Autodesk Inventor part; units mm, degrees
ref_plane "YZ Plane" through (0, 0, 0) normal (1, 0, 0) x (0, 1, 0)
ref_plane "XZ Plane" through (0, 0, 0) normal (0, 1, 0) x (-1, 0, 0)
ref_plane "XY Plane" through (0, 0, 0) normal (0, 0, 1) x (1, 0, 0)
sketch "Sketch1" plane through (0, 0, 0) normal (0, 1, 0) x (-1, 0, 0)
  line L0 (0, 0) -> (10.922, 0)
  line L1 (10.922, 0) -> (10.922, 203.2)
  line L2 (10.922, 203.2) -> (0, 203.2)
  line L3 (0, 203.2) -> (0, 0)
  line L4 (10.922, 203.2) -> (-166.878, 203.2)
  line L5 (-166.878, 203.2) -> (-166.878, 181.102)
  line L6 (-166.878, 181.102) -> (10.922, 181.102)
  line L7 (10.922, 181.102) -> (10.922, 203.2)
  point P0 (0, 181.102)
  dimension "d0" = 10.922
  dimension "d1" = 203.2
  dimension "d16" = 177.8
  dimension "d17" = 22.098
extrude "Extrusion1" add sketch "Sketch1" along normal blind 50.8
sketch "Sketch3" plane through (0, 0, 181.102) normal (1, 0, 0) x (0, 0, -1)
  circle A0 centre (28.702, 25.4) radius 2.5797
  circle A1 centre (130.302, 25.4) radius 2.5797
  line L0 (181.102, 0) -> (181.102, 50.8)
  line L1 (0, 0) -> (181.102, 0)
  circle A2 centre (130.302, 25.4) radius 3.9688
  circle A3 centre (28.702, 25.4) radius 3.9687
  dimension "d18" = 5.1594
  dimension "d19" = 5.1594
  dimension "d20" = 0
  dimension "d21" = 101.6
  dimension "d22" = 50.8
  dimension "d23" = 25.4
  dimension "d24" = 7.9375
  dimension "d25" = 7.9375
sketch "Sketch4" plane through (166.878, 0, 181.102) normal (0, 0, -1) x (-1, 0, 0)
  circle A0 centre (50.8, 25.4) radius 2.5797
  circle A1 centre (127, 25.4) radius 2.5797
  line L0 (0, 0) -> (0, 50.8)
  circle A2 centre (50.8, 25.4) radius 3.9687
  circle A3 centre (127, 25.4) radius 3.9687
  line L1 (0, 0) -> (166.878, 0)
  dimension "d26" = 5.1594
  dimension "d27" = 5.1594
  dimension "d28" = 0
  dimension "d29" = 76.2
  dimension "d30" = 50.8
  dimension "d31" = 7.9375
  dimension "d32" = 7.9375
  dimension "d33" = 25.4
extrude "Extrusion4" cut sketch "Sketch4" against normal through all contours A0 | A1
extrude "Extrusion5" cut sketch "Sketch4" against normal blind 5.1594 contours A0 | A1 | A2 | A3
extrude "Extrusion6" cut sketch "Sketch3" against normal blind 5.1594 contours A0 | A1 | A2 | A3
extrude "Extrusion7" cut sketch "Sketch3" against normal through all contours A0 | A1
equation "\"d19\" = d18"
equation "\"d26\" = d18"
equation "\"d27\" = d26"
equation "\"d31\" = d24"
equation "\"d32\" = d31"
properties part number "battery shim"
The listing builds one solid part. Answer for the finished solid, in the listing's coordinates (mm). A direction names the side the tool comes from. Coordinates: 2 decimals unless noted, no trailing zeros. Write each loop counter-clockwise with the first axis right and the second up, starting at its lowest first coordinate (ties: lowest second). Pieces come first, ordered by that corner, then holes. Notation, with made-up numbers: (-20, 77.5) - (1, 77.5) arc R21 cw to (1, 86.5) - close; hole circle Ø9 at (25, 34.5). An arc over 180 degrees is marked (long way). Return JSON: item names as keys, results as strings. Group by question number.
1. Straight lines are drawn through the part: L1, parallel to Z at x = -2, y = 25; L2, parallel to X at y = 25, z = 184; L3, parallel to X at y = 25, z = 199. For each, find the intervals that lie inside material, in ascending order.
2. A cutting plane is placed at A-A, the plane z = 50.8. Determine the outline of the cut face in (x, y).
3. Which of the six approach directions +Z, -Z, +X, -X, +Y, -Y give full straight-line access (tool end or side, diameter ignored) to faces 4 (the flat face through (-5, 25, 0)), 5 (the cylindrical face through (118.655, 25.513, 194.612)), 6 (the flat face through (85, 25, 181.102)), 7 (the cylindrical face through (-2.544, 25.575, 54.765)), 8 (the flat face through (113, 25, 186.261))?
4. A cutting plane is placed at D-D, the plane y = 44.5. Determine the outline of the cut face in (x, z), plus the area to 3 significant figures.
5. Given pin 1 (6 mm diameter, centred on y = 25.4, z = 152.4, fed in from +X); pin 2 (6 mm diameter, centred on x = 39.878, y = 25.4, fed in from -Z); pin 3 (15 mm diameter, centred on x = 115.5, y = 27.5, fed in from -Z), each flat-ended and moving along its own axis, determine where each tip first touches the part or whether it passes through.
6. Determine the mould class of faces 1 (the flat face through (45, 50.8, 185)), 2 (the flat face through (0, 25, 92)), 3 (the cylindrical face through (37.5, 24.4, 194.6)) for opening direction X: released by +X, released by -X, zero draft, split by the parting line, or undercut.
7. A cutting plane is placed at C-C, the plane y = 25.4. Give the number of separate pieces and of enclosed holes in the cut face, plus the area to 3 significant figures.
Ans:
{
 "1": {"L1": "0 to 46.85, 54.75 to 148.45, 156.35 to 203.2", "L2": "-10.92 to 35.93, 43.83 to 112.13, 120.03 to 166.88", "L3": "-10.92 to 37.33, 42.43 to 113.53, 118.63 to 166.88"},
 "2": {"outline": "(-10.92, 0) - (0, 0) - (0, 21.43) - (-5.16, 21.43) - (-5.16, 22.82) - (-10.92, 22.82) - close; (-10.92, 27.98) - (-5.16, 27.98) - (-5.16, 29.37) - (0, 29.37) - (0, 50.8) - (-10.92, 50.8) - close"},
 "3": {"face 4": "-Z, +X, -X, +Y, -Y", "face 5": "+Z, -Z", "face 6": "-Z, +X, +Y, -Y", "face 7": "+X", "face 8": "-Z"},
 "4": {"outline": "(-10.92, 0) - (0, 0) - (0, 181.1) - (166.88, 181.1) - (166.88, 203.2) - (-10.92, 203.2) - close", "area": "5,910 mm²"},
 "5": {"pin 1": "x = -5.16", "pin 2": "z = 186.26", "pin 3": "z = 181.1"},
 "6": {"face 1": "zero draft", "face 2": "released by +X", "face 3": "undercut"},
 "7": {"separate pieces": "5", "enclosed holes": "0", "area": "5,510 mm²"}
}
